Part model, mm, in its own coordinate system. Face numbers are marked on the shaded views. A direction names the side the tool comes from. Round coordinates to 2 decimals unless told otherwise and drop trailing zeros. Write each loop counter-clockwise with the first axis right and the second up, starting at its lowest first coordinate (ties: lowest second). Pieces come first, ordered by that corner, then holes.
1) Saw through at B-B on x = -12.5. Write the cut outline in (y, z), and give its area (3 significant figures).
2) Saw through at A-A on y = 8.75. Write the cut outline in (x, z).
3) Flat gauge pins, fed straight in: pin 1 (2 mm diameter, centred on y = -12.5, z = 1, fed in from -X); pin 2 (0.5 mm diameter, centred on x = 2, z = 2.5, fed in from -Y); pin 3 (0.9 mm diameter, centred on x = -2, z = 2, fed in from +Y). Where does each tip first touch, or does it go through?
4) Saw through at C-C on y = 3. Write the cut outline in (x, z).
5) Pull direction X, two halves, no side cores. Call the marked faces 6, 7, 8 and 9: +X half, -X half, draft (parallel to the pull), parting line (faces both ways), or undercut.
6) Saw through at D-D on z = 3.3. Count the separate pieces of the cut face and the enclosed holes in it, and give its area (3 significant figures).
7) Which spindle directions (+Z, -Z, +X, -X, +Y, -Y) get a long thin tool onto all of the face, cutting with end or side? Do the marked faces 1, 2, 3, 4 and 5. Say none if no direction does.
8) Drill centre lines: L1, parallel to X at y = -10.75, z = 1.4; L2, parallel to Y at x = -12.5, z = 2.05; L3, parallel to X at y = 7.75, z = 0.85. Where is each one in solid material? Low to high.
Autodesk Inventor part; units mm, degrees
ref_plane "YZ Plane" through (0, 0, 0) normal (1, 0, 0) x (0, 1, 0)
ref_plane "XZ Plane" through (0, 0, 0) normal (0, 1, 0) x (-1, 0, 0)
ref_plane "XY Plane" through (0, 0, 0) normal (0, 0, 1) x (1, 0, 0)
sketch "Эскиз1" plane through (0, 0, 0) normal (0, 0, 1) x (1, 0, 0)
  line L0 (20, 9.6) -> (-20, 9.6)
  line L1 (-20, 9.6) -> (-20, -9.6)
  line L2 (-20, -9.6) -> (20, -9.6)
  line L3 (20, -9.6) -> (20, 9.6)
  line L4 (20, 9.6) -> (-20, -9.6) construction
  line L5 (-20, 9.6) -> (20, -9.6) construction
  line L6 (-16, 9.6) -> (-8, 9.6)
  line L7 (-8, 9.6) -> (-8, 13.6)
  line L8 (-8, 13.6) -> (-16, 13.6)
  line L9 (-16, 13.6) -> (-16, 9.6)
  line L10 (16, 9.6) -> (8, 9.6)
  line L11 (8, 9.6) -> (8, 13.6)
  line L12 (8, 13.6) -> (16, 13.6)
  line L13 (16, 13.6) -> (16, 9.6)
  line L14 (-16, -9.6) -> (-8, -9.6)
  line L15 (-8, -9.6) -> (-8, -13.6)
  line L16 (-8, -13.6) -> (-16, -13.6)
  line L17 (-16, -13.6) -> (-16, -9.6)
  line L18 (8, -9.6) -> (16, -9.6)
  line L19 (16, -9.6) -> (16, -13.6)
  line L20 (16, -13.6) -> (8, -13.6)
  line L21 (8, -13.6) -> (8, -9.6)
  point P0 (0, 0)
  point P1 (-16, 11.6)
  point P2 (16, -9.6)
  point P3 (8, 9.6)
  point P4 (-8, 9.6)
  dimension "d0" = 40
  dimension "d1" = 19.2
  dimension "d2" = 8
  dimension "d3" = 4
  dimension "d4" = 8
  dimension "d5" = 4
  dimension "d6" = 4
  dimension "d7" = 4
  dimension "d8" = 8
  dimension "d9" = 4
extrude "Выдавливание1" add sketch "Эскиз1" along normal blind 4
sketch "Эскиз2" plane through (0, 0, 4) normal (0, 0, 1) x (1, 0, 0)
  line L0 (8, 9.6) -> (-8, 9.6)
  line L1 (-1.7, 9.6) -> (1.7, 9.6)
  line L2 (1.7, 9.6) -> (1.7, 3.6)
  line L3 (1.7, 3.6) -> (-1.7, 3.6)
  line L4 (-1.7, 3.6) -> (-1.7, 9.6)
  line L5 (0, 9.6) -> (0, 3.6) construction
  line L6 (-2.8, 5.2) -> (2.8, 5.2)
  line L7 (2.8, 5.2) -> (2.8, 7.6)
  line L8 (2.8, 7.6) -> (-2.8, 7.6)
  line L9 (-2.8, 7.6) -> (-2.8, 5.2)
  line L10 (-2.8, 5.2) -> (2.8, 7.6) construction
  line L11 (2.8, 5.2) -> (-2.8, 7.6) construction
  line L12 (-20, 9.6) -> (-20, -9.6)
  line L13 (-20, 0) -> (20, 0) construction
  line L14 (20, -9.6) -> (20, 9.6)
  line L15 (8, -9.6) -> (-8, -9.6)
  line L16 (-1.7, -9.6) -> (1.7, -9.6)
  line L17 (1.7, -9.6) -> (1.7, -3.6)
  line L18 (1.7, -3.6) -> (-1.7, -3.6)
  line L19 (-1.7, -3.6) -> (-1.7, -9.6)
  line L20 (0, -9.6) -> (0, -3.6) construction
  line L21 (-2.8, -5.2) -> (2.8, -5.2)
  line L22 (2.8, -5.2) -> (2.8, -7.6)
  line L23 (2.8, -7.6) -> (-2.8, -7.6)
  line L24 (-2.8, -7.6) -> (-2.8, -5.2)
  line L25 (-2.8, -5.2) -> (2.8, -7.6) construction
  line L26 (2.8, -5.2) -> (-2.8, -7.6) construction
  point P0 (0, 0)
  point P1 (0, 6.4)
  point P2 (0, -6.4)
  point P3 (1.7, 5.2)
  point P4 (1.7, 7.6)
  point P5 (1.7, 9.6)
  point P6 (-1.7, 7.6)
  point P7 (-1.7, 5.2)
  point P8 (-1.7, -7.6)
  point P9 (1.7, -7.6)
  point P10 (1.7, -5.2)
  point P11 (-1.7, -5.2)
  dimension "d12" = 3.4
  dimension "d13" = 6
  dimension "d14" = 5.6
  dimension "d15" = 2.4
  dimension "d16" = 2
extrude "Выдавливание2" cut sketch "Эскиз2" against normal blind 10
sketch "Эскиз3" plane through (0, 0, 0) normal (0, 0, -1) x (-1, 0, 0)
  circle A0 centre (12.5, 3) radius 1.6
  circle A1 centre (-12.5, 3) radius 1.6
  point P0 (0, 0)
extrude "Выдавливание3" cut sketch "Эскиз3" against normal blind 10
properties part number "стена_каретки"
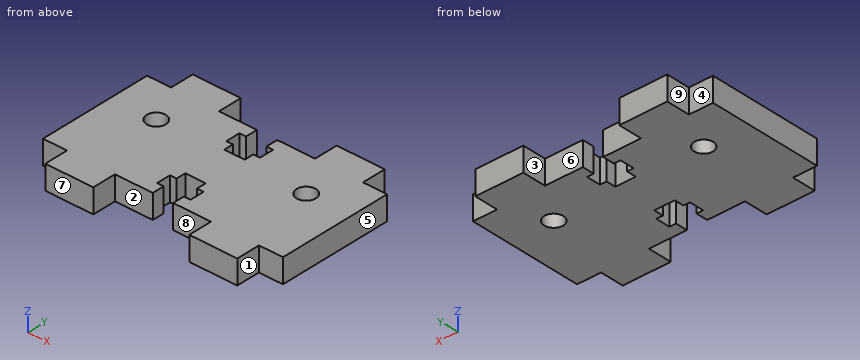
Completed:
1. outline: (-13.6, 0) - (1.4, 0) - (1.4, 4) - (-13.6, 4) - close; (4.6, 0) - (13.6, 0) - (13.6, 4) - (4.6, 4) - close
1. area: 96.0 mm2
2. outline: (-20, 0) - (-1.7, 0) - (-1.7, 4) - (-20, 4) - close; (1.7, 0) - (20, 0) - (20, 4) - (1.7, 4) - close
3. pin 1: stops at x = -16
3. pin 2: stops at y = -9.6
3. pin 3: stops at y = 9.6
4. outline: (-20, 0) - (-14.1, 0) - (-14.1, 4) - (-20, 4) - close; (-10.9, 0) - (10.9, 0) - (10.9, 4) - (-10.9, 4) - close; (14.1, 0) - (20, 0) - (20, 4) - (14.1, 4) - close
5. face 6: undercut
5. face 7: draft
5. face 8: undercut
5. face 9: -X half
6. separate pieces: 1
6. enclosed holes: 2
6. area: 829 mm2
7. face 1: +Z, -Z, +X, -Y
7. face 2: +Z, -Z, -Y
7. face 3: +Z, -Z, +Y
7. face 4: +Z, -Z, -X, +Y
7. face 5: +Z, -Z, +X, +Y, -Y
8. L1: x = -16 to -8, 8 to 16
8. L2: y = -13.6 to 1.4, 4.6 to 13.6
8. L3: x = -20 to -1.7, 1.7 to 20
